Verification items for this drawing (mm, ordinates from the low corner). Coordinates: 2 decimals unless noted, no trailing zeros. Write each loop counter-clockwise with the first axis right and the second up, starting at its lowest first coordinate (ties: lowest second). Pieces come first, ordered by that corner, then holes. Notation, with made-up numbers: (44, 46) -> (77, 46) arc R19 cw to (77, 62) -> close; hole circle Ø10 at (77, 67). An arc over 180 degrees is marked (long way). One line per question, with ' | ' between items.
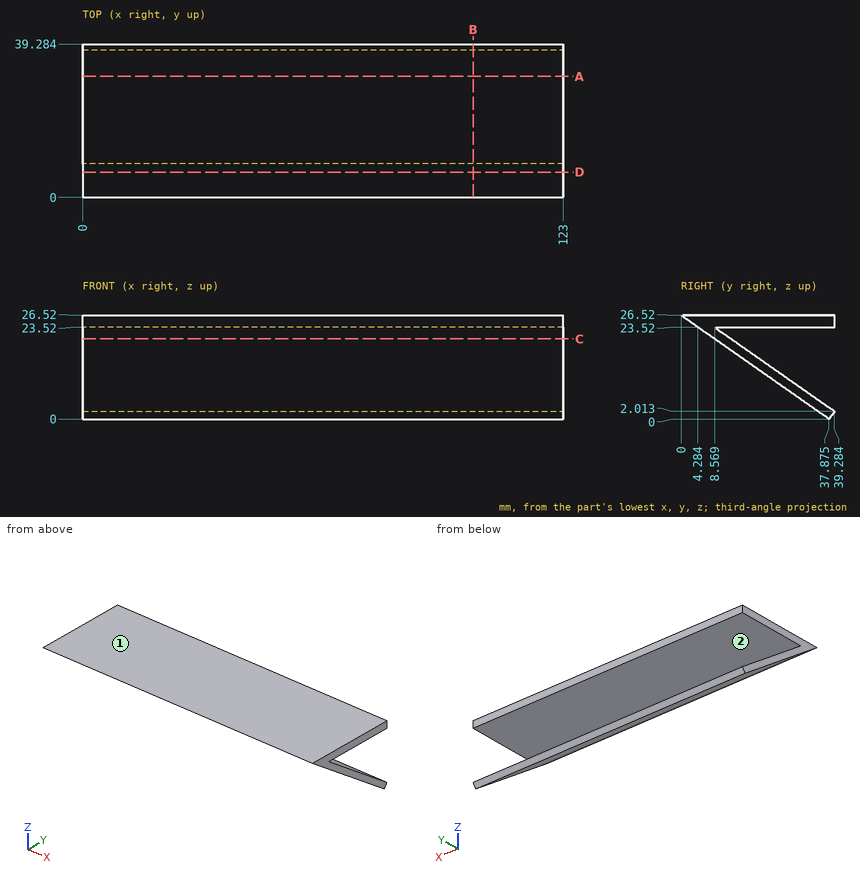
(1) Depth check by flat-ended pin: P1, Ø1.5, axis at x = 28.5, z = 4, coming from the -Y side; P2, Ø3, axis at x = 46, y = 19.5, coming from the -Z side (1 decimal); P3, Ø3, axis at x = 56, z = 16.5, coming from the -Y side; P4, Ø1, axis at y = 22, z = 14, coming from the -X side. Enter the tip coordinate at first touch or a pass-through.
Answers below:
P1: stops at y = 31.09 | P2: stops at z = 11.8 | P3: stops at y = 12.17 | P4: stops at x = 0
(2) Cross-section at B-B (x = 100). Record the cut outline in (y, z) (1 decimal), plus the area to 3 significant figures.
Answers below:
outline: (0, 26.5) -> (37.9, 0) -> (39.3, 2) -> (8.6, 23.5) -> (39.3, 23.5) -> (39.3, 26.5) -> close | area: 208 mm²
(3) Material ranges on line 1 (Z direction, x = 43.5, y = 17.5) (1 decimal); line 2 (Z direction, x = 71, y = 20) (1 decimal); line 3 (Y direction, x = 58.5, z = 18.5) (1 decimal), recorded low to high.
Answers below:
line 1: z = 14.3 to 17.3, 23.5 to 26.5 | line 2: z = 12.5 to 15.5, 23.5 to 26.5 | line 3: y = 11.5 to 15.7
(4) Cross-section at D-D (y = 6.5). Record the cut outline in (x, z).
Answers below:
outline: (0, 21.97) -> (123, 21.97) -> (123, 26.52) -> (0, 26.52) -> close
(5) Cross-section at C-C (z = 20.5). Record the cut outline in (x, y), plus the area to 3 significant figures.
Answers below:
outline: (0, 8.6) -> (123, 8.6) -> (123, 12.88) -> (0, 12.88) -> close | area: 527 mm²
(6) Draft check along Z on the marked faces 1 and 2. Enter one of: pulls with the +Z half, pulls with the -Z half, needs draft (parallel to the pull), parting line crosses it, or undercut.
Answers below:
face 1: pulls with the +Z half | face 2: undercut
(7) Cross-section at A-A (y = 31). Record the cut outline in (x, z).
Answers below:
outline: (0, 4.81) -> (123, 4.81) -> (123, 7.81) -> (0, 7.81) -> close; (0, 23.52) -> (123, 23.52) -> (123, 26.52) -> (0, 26.52) -> close
